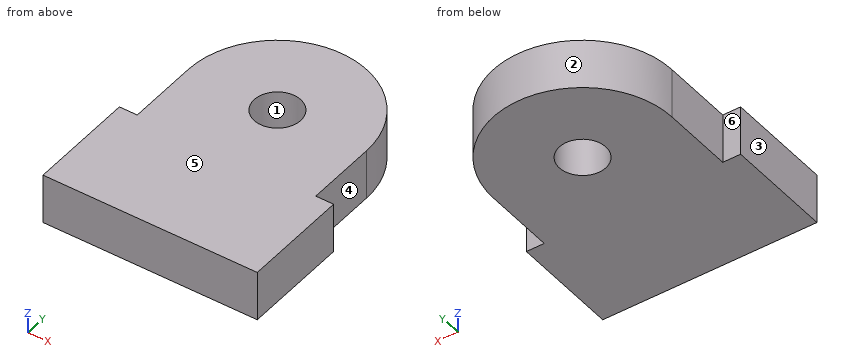
from build123d import *

# Parameters (mm, degrees)
Y_KSEKLIK_EKSTR_ZYON1_DEPTH = 7
IZIM4_R                     = 3.25
KES_EKSTR_ZYON1_DEPTH       = 30.983328701


with BuildPart() as part:
    # Çizim1 → Yükseklik-Ekstrüzyon1 (new body)
    with BuildSketch(Plane.XY):
        with BuildLine():
            Line((-12.5, 0), (-12.5, -10))
            Line((-12.5, -10), (-15, -10))
            Line((-15, -10), (-15, -25))
            Line((-15, -25), (15, -25))
            Line((15, -25), (15, -10))
            Line((15, -10), (12.5, -10))
            Line((12.5, -10), (12.5, 0))
            ThreePointArc((12.5, 0), (0, 12.5), (-12.5, 0))
        make_face()
    extrude(amount=Y_KSEKLIK_EKSTR_ZYON1_DEPTH)

    # Çizim4 → Kes-Ekstrüzyon1 (cut, through all)
    with BuildSketch(Plane.XY.offset(7)):
        Circle(IZIM4_R)
    extrude(amount=-KES_EKSTR_ZYON1_DEPTH, mode=Mode.SUBTRACT)


solid = part.part
Read the model definition and answer for the solid it produces. Units are mm, in the model's axes. Face numbers are marked on the shaded views. A direction names the side the tool comes from. Give positions to 0.01 mm unless a question says otherwise; leave off trailing zeros. Write each loop counter-clockwise with the first axis right and the second up, starting at its lowest first coordinate (ties: lowest second). Pieces come first, ordered by that corner, then holes. Notation, with made-up numbers: M 70.25,-4.75 L 119.25,-4.75 A5 ccw 119.25,0.25 Z; hole C -4,26.25 d7. An arc over 180 degrees is marked long. One line per item, written item: value. Start each with the question number.
(1) Find the intervals of material crossed by line 1 (Y direction, x = 0, z = 3); line 2 (X direction, y = -7, z = 5.75); line 3 (Y direction, x = -13, z = 1), in increasing order.
(2) Find section B-B (z = 3.5). Determine the outline of the cut face in (x, y).
(3) Find section A-A (x = 0). Determine the outline of the cut face in (y, z).
(4) Find section D-D (x = -9). Determine the outline of the cut face in (y, z).
(5) Find section C-C (x = 8.5). Determine the outline of the cut face in (y, z).
(6) Flat-ended cylindrical pins translate along their axes: pin 1 Ø1.2 at (x, z) = (14, 2) entering from +Y; pin 2 Ø1.5 at (y, z) = (-8.5, 3) entering from -X; pin 3 Ø3.5 at (y, z) = (-2.5, 2.5) entering from +X. Find the tip coordinate at first contact, or state that the pin passes through.
(7) A tool of negligible diameter and unlimited length cuts with its end or side. For the marked faces 5 and 6, from which of +Z, -Z, +X, -X, +Y, -Y can it reach the whole face along a straight path? Write none if from no direction.
(8) Determine the mould class of the marked faces 1, 2, 3 and 4 for opening direction X: pulls with the +X half, pulls with the -X half, needs draft (parallel to the pull), parting line crosses it, or undercut.
Results below:
1. line 1: y = -25 to -3.25, 3.25 to 12.5
1. line 2: x = -12.5 to 12.5
1. line 3: y = -25 to -10
2. outline: M -15,-25 L 15,-25 L 15,-10 L 12.5,-10 L 12.5,0 A12.5 ccw -12.5,0 L -12.5,-10 L -15,-10 Z; hole C 0,0 d6.5
3. outline: M -25,0 L -3.25,0 L -3.25,7 L -25,7 Z; M 3.25,0 L 12.5,0 L 12.5,7 L 3.25,7 Z
4. outline: M -25,0 L 8.67,0 L 8.67,7 L -25,7 Z
5. outline: M -25,0 L 9.17,0 L 9.17,7 L -25,7 Z
6. pin 1: stops at y = -10
6. pin 2: stops at x = -12.5
6. pin 3: stops at x = 12.5
7. face 5: +Z, +X, -X, +Y, -Y
7. face 6: +Z, -Z, -X, +Y
8. face 1: undercut
8. face 2: parting line crosses it
8. face 3: pulls with the -X half
8. face 4: pulls with the +X half
